For this review, take the finished solid that the model builds, in its own axes (mm). A direction names the side the tool comes from. Round coordinates to 2 decimals unless told otherwise and drop trailing zeros. Write each loop counter-clockwise with the first axis right and the second up, starting at its lowest first coordinate (ties: lowest second). Pieces come first, ordered by that corner, then holes. Notation, with made-up numbers: (69.25, -33) - (82.25, -33) arc R20 cw to (82.25, 1) - close; hole circle Ø3 at (61.25, -12.5). An arc over 180 degrees is marked (long way). Answer in a Markdown table with one row per item. Add a question column.
from build123d import *

# Parameters (mm, degrees)
SKETCH2_R               = 34.8615
SKETCH2_R_2             = 33.528
BOSS_EXTRUDE1_DEPTH     = 25.4
BOSS_EXTRUDE2_START     = 50.8
SKETCH3_R               = 34.8615
BOSS_EXTRUDE2_DEPTH     = 50.8
SKETCH4_R               = 31.75
CUT_EXTRUDE2_DEPTH      = 94.044402901
SKETCH6_R               = 31.75
CUT_EXTRUDE4_DEPTH      = 50.8
CUT_EXTRUDE5_REACH      = 95.044
CUT_EXTRUDE5_END_RADIUS = 31.75
SKETCH7_R               = 10.16


with BuildPart() as part:
    # Sketch2 → Boss-Extrude1 (new body)
    with BuildSketch(Plane.XY):
        Circle(SKETCH2_R)
        Circle(SKETCH2_R_2, mode=Mode.SUBTRACT)
    extrude(amount=BOSS_EXTRUDE1_DEPTH)

    # Sketch3 → Boss-Extrude2 (add)
    with BuildSketch(Plane(origin=(0, 0, 0), x_dir=(-1, 0, 0), z_dir=(0, 0, -1)).offset(BOSS_EXTRUDE2_START)):
        Circle(SKETCH3_R)
    extrude(amount=-BOSS_EXTRUDE2_DEPTH)

    # Sketch4 → Cut-Extrude2 (cut, through all)
    with BuildSketch(Plane(origin=(34.8615, 0, 0), x_dir=(0, 0, -1), z_dir=(1, 0, 0))):
        with Locations((57.15, 0)):
            Circle(SKETCH4_R)
    extrude(amount=-CUT_EXTRUDE2_DEPTH, mode=Mode.SUBTRACT)

    # Sketch6 → Cut-Extrude4 (cut)
    with BuildSketch(Plane.XY):
        Circle(SKETCH6_R)
    extrude(amount=-CUT_EXTRUDE4_DEPTH, mode=Mode.SUBTRACT)

    # Cut-Extrude5: up to this cylinder (the profile starts outside it)
    cut_extrude5_end = Plane(origin=(0, 0, -16.51), z_dir=(0, 0, 1)) * Cylinder(CUT_EXTRUDE5_END_RADIUS, 254.588, mode=Mode.PRIVATE)
    # Sketch7 → Cut-Extrude5 (cut, up to the surface)
    with BuildSketch(Plane(origin=(0, 34.8615, 0), x_dir=(-1, 0, 0), z_dir=(0, 1, 0)), mode=Mode.PRIVATE) as cut_extrude5_sk1:
        with Locations(Location((0, -16.51, 0), (0, 0, 90))):
            Circle(SKETCH7_R)
    cut_extrude5_tool1 = extrude(cut_extrude5_sk1.sketch, amount=-CUT_EXTRUDE5_REACH, mode=Mode.PRIVATE) - cut_extrude5_end
    add(cut_extrude5_tool1.solids().sort_by_distance((0, 34.8615, -16.51))[0], mode=Mode.SUBTRACT)


solid = part.part
Q1. Add section A-A on y = 0. State the section outline as (x, z) points.
Q2. To check wall thickness, follow probe 1 along Y at (x, z) = (0, 6.5); probe 2 along Y at (x, z) = (1, 1); probe 3 along X at (y, z) = (-13.5, -18). State the ranges of each line that lie inside material, in increasing order.
Q3. Add section D-D on z = -1. State the section outline as (x, y) points, then the cut area to 3 significant figures.
Q4. Insertion check: pin 1 Ø2 at (x, z) = (-18, -2) entering from -Y; pin 2 Ø5 at (y, z) = (-20, 16.5) entering from +X; pin 3 Ø12 at (x, z) = (0, -16.51) entering from -Y. Each pin has a flat end and moves straight along its axis. Give the tip position at first contact, or say it passes through.
Q5. Add section B-B on x = 0. State the section outline as (y, z) points.
Q6. Add section C-C on x = -28.5. State the section outline as (y, z) points.
Q7. Tool access review of faces 3 (the face through (0.45, 32.5, -26.66)), 4 (the face through (-6.883, -30.995, -19.4)), 5 (the face through (32, 10, 13)): name each direction out of +Z, -Z, +X, -X, +Y, -Y from which nothing blocks a thin tool from reaching the whole face with its end or side.
Q8. Draft analysis for pull direction Y (two halves, no side actions). For faces 1 (the face through (0, 33, -50.8)), 2 (the face through (31.237, 6.596, -26.093)), state which applies: released by +Y, released by -Y, zero draft, split by the parting line, or undercut.
Answer sheet:
| question | item | result |
|---|---|---|
| 1 | outline | (-34.86, -25.4) - (-31.75, -25.4) - (-31.75, 0) - (-33.53, 0) - (-33.53, 25.4) - (-34.86, 25.4) - close; (31.75, -25.4) - (34.86, -25.4) - (34.86, 25.4) - (33.53, 25.4) - (33.53, 0) - (31.75, 0) - close |
| 2 | probe 1 | y = -34.86 to -33.53, 33.53 to 34.86 |
| 2 | probe 2 | y = -34.85 to -33.51, 33.51 to 34.85 |
| 2 | probe 3 | x = -32.14 to -28.74, 28.74 to 32.14 |
| 3 | outline | circle Ø69.72 at (0, 0); hole circle Ø63.5 at (0, 0) |
| 3 | area | 651 mm² |
| 4 | pin 1 | stops at y = -30.44 |
| 4 | pin 2 | stops at x = 30.15 |
| 4 | pin 3 | stops at y = -34.86 |
| 5 | outline | (-34.86, -50.8) - (-31.75, -50.8) - (-31.75, 0) - (-33.53, 0) - (-33.53, 25.4) - (-34.86, 25.4) - close; (31.75, -50.8) - (34.86, -50.8) - (34.86, -26.67) - (31.75, -26.67) - close; (31.75, -6.35) - (34.86, -6.35) - (34.86, 25.4) - (33.53, 25.4) - (33.53, 0) - (31.75, 0) - close |
| 6 | outline | (-20.08, -32.55) arc R31.75 cw to (-13.99, -28.65) - (-13.99, 0) - (-17.66, 0) - (-17.66, 25.4) - (-20.08, 25.4) - close; (13.99, -28.65) arc R31.75 cw to (20.08, -32.55) - (20.08, 25.4) - (17.66, 25.4) - (17.66, 0) - (13.99, 0) - close |
| 7 | face 3 | +Y |
| 7 | face 4 | +Z, -Z |
| 7 | face 5 | +Z |
| 8 | face 1 | zero draft |
| 8 | face 2 | undercut |
